Build history of the part. All positions in model axes, mm. Face numbers are marked on the shaded views. A direction names the side the tool comes from. Round coordinates to 2 decimals unless told otherwise and drop trailing zeros. Loops run counter-clockwise (first coordinate to the right, second up) from the corner with the lowest first, then second, coordinate; pieces in that order, holes last. Notation, with made-up numbers: (16.25, 63) - (65.25, 63) arc R28 cw to (65.25, 88) - close; hole circle Ø10 at (-4.75, 42). An arc over 180 degrees is marked (long way). Put each result on its own line as item: value. Start each with the question number.
from build123d import *

# Parameters (mm, degrees)
BOSS_EXTRUDE1_DEPTH = 412.75
SKETCH2_R           = 2.5796875
CUT_EXTRUDE1_DEPTH  = 417.844974931
SKETCH3_R           = 2.5796875
CUT_EXTRUDE2_DEPTH  = 417.60307323


with BuildPart() as part:
    # Sketch1 → Boss-Extrude1 (new body)
    with BuildSketch(Plane.XY):
        with BuildLine():
            Line((0, 0), (0, 50.8))
            Line((0, 50.8), (6.35, 50.8))
            Line((6.35, 50.8), (6.35, 12.7))
            ThreePointArc((6.35, 12.7), (8.209871939, 8.209871939), (12.7, 6.35))
            Line((12.7, 6.35), (34.925, 6.35))
            Line((34.925, 6.35), (34.925, 0))
            Line((34.925, 0), (0, 0))
        make_face()
    extrude(amount=BOSS_EXTRUDE1_DEPTH)

    # Sketch2 → Cut-Extrude1 (cut, through all)
    with BuildSketch(Plane(origin=(6.35, 0, 0), x_dir=(0, 0, -1), z_dir=(1, 0, 0))):
        with Locations(Location((-374.015, 27.0002, 0), (0, 0, 90))):
            Circle(SKETCH2_R)
        with Locations(Location((-38.735, 26.9875, 0), (0, 0, 90))):
            Circle(SKETCH2_R)
    extrude(amount=-CUT_EXTRUDE1_DEPTH, mode=Mode.SUBTRACT)

    # Sketch3 → Cut-Extrude2 (cut, through all)
    with BuildSketch(Plane(origin=(0, 6.35, 0), x_dir=(1, 0, 0), z_dir=(0, 1, 0))):
        with Locations(Location((25.146, -373.38, 0), (0, 0, 180))):
            Circle(SKETCH3_R)
        with Locations(Location((25.146, -39.37, 0), (0, 0, 180))):
            Circle(SKETCH3_R)
    extrude(amount=-CUT_EXTRUDE2_DEPTH, mode=Mode.SUBTRACT)


solid = part.part
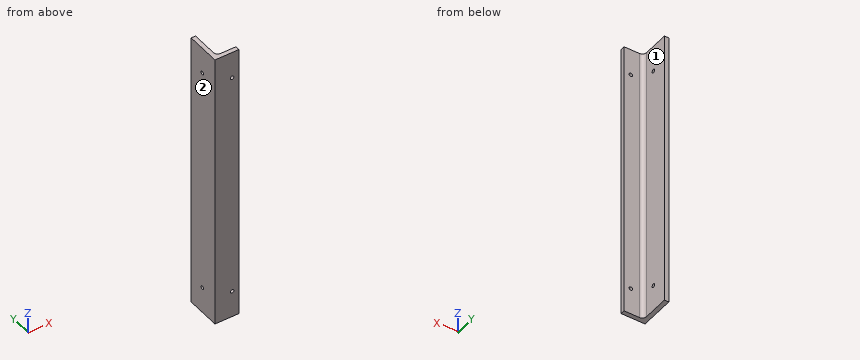
Item 1: Slice it at A-A (z = 287). Give the cut face in (x, y) (3 decimals).
Item 2: Drop flat-ended pins along their axis: pin 1 Ø4 at (y, z) = (29, 91.5) entering from +X; pin 2 Ø1 at (y, z) = (12.5, 105) entering from +X; pin 3 Ø11 at (x, z) = (24.5, 257.5) entering from +Y. Give the stop position or say it passes through.
Item 3: Which spindle directions (+Z, -Z, +X, -X, +Y, -Y) get a long thin tool onto all of the face, cutting with end or side? Do the marked faces 1 and 2. Say none if no direction does.
Item 4: Slice it at B-B (y = 42.5). Give the cut face in (x, z), plus the area to 3 significant figures.
Item 5: Drill centre lines: probe 1 along X at (y, z) = (5, 39) (3 decimals); probe 2 along Y at (x, z) = (30.5, 319). Where is each one in solid material? Low to high. Write a range as [from, to].
Computed values:
1. outline: (0, 0) - (34.925, 0) - (34.925, 6.35) - (12.7, 6.35) arc R6.35 cw to (6.35, 12.7) - (6.35, 50.8) - (0, 50.8) - close
2. pin 1: stops at x = 6.35
2. pin 2: stops at x = 6.39
2. pin 3: stops at y = 6.35
3. face 1: +Z, -Z, +X, +Y
3. face 2: +Z, -Z, -X, +Y, -Y
4. outline: (0, 0) - (6.35, 0) - (6.35, 412.75) - (0, 412.75) - close
4. area: 2,620 mm^2
5. probe 1: x = [0, 22.593], [27.699, 34.925]
5. probe 2: y = [0, 6.35]
